Check sheet for the modelled part. Datum: model origin and axes. Units: mm. A direction names the side the tool comes from. Give positions to 0.01 mm unless a question says otherwise; leave off trailing zeros. Write each loop counter-clockwise with the first axis right and the second up, starting at its lowest first coordinate (ties: lowest second). Pieces come first, ordered by that corner, then holes. Notation, with made-up numbers: (36, 79.25) - (94, 79.25) arc R26 ccw to (94, 102.25) - close; hole circle Ø11 at (35, 45.25). An arc over 180 degrees is marked (long way). Return JSON: item names as keys, results as strings. Group by question number.
```python
from build123d import *

# Parameters (mm, degrees)
ESQUISSE1_W        = 29.5
ESQUISSE1_H        = 13
BOSS_EXTRU_2_DEPTH = 7.2
ESQUISSE2_W        = 29.5
ESQUISSE2_H        = 8.4
BOSS_EXTRU_3_DEPTH = 4.3
ESQUISSE4_W        = 7.5
ESQUISSE4_H        = 7.2
BOSS_EXTRU_4_DEPTH = 2
ESQUISSE8_W        = 10.1
ESQUISSE8_H        = 5.9
BOSS_EXTRU_5_DEPTH = 1.2
BOSS_EXTRU_6_START = -10.1
BOSS_EXTRU_6_DEPTH = 10.1
ESQUISSE10_R       = 1.6
BOSS_EXTRU_8_DEPTH = 2


with BuildPart() as part:
    # Esquisse1 → Boss.-Extru.2 (new body)
    with BuildSketch(Plane.XY):
        Rectangle(ESQUISSE1_W, ESQUISSE1_H)
    extrude(amount=BOSS_EXTRU_2_DEPTH)

    # Esquisse2 → Boss.-Extru.3 (add)
    with BuildSketch(Plane.XY.offset(7.2)):
        Rectangle(ESQUISSE2_W, ESQUISSE2_H)
    extrude(amount=BOSS_EXTRU_3_DEPTH)

    # Esquisse4 → Boss.-Extru.4 (add)
    with BuildSketch(Plane.XY.offset(11.5)):
        with Locations((-10.25, 0)):
            Rectangle(ESQUISSE4_W, ESQUISSE4_H)
    extrude(amount=BOSS_EXTRU_4_DEPTH)

    # Esquisse8 → Boss.-Extru.5 (add)
    with BuildSketch(Plane.XY.offset(3.3)):
        with Locations((0, -9.45)):
            Rectangle(ESQUISSE8_W, ESQUISSE8_H)
    extrude(amount=BOSS_EXTRU_5_DEPTH)

    # Esquisse9 → Boss.-Extru.6 (add)
    with BuildSketch(Plane(origin=(5.05, 0, 0), x_dir=(0, 0, -1), z_dir=(1, 0, 0)).offset(BOSS_EXTRU_6_START)):
        Polygon((-4.5, -12.4), (-10.0771346, -12.4), (-10.0771346, -6.830479263), (-8.508865165, -6.830479263), (-7.2, -5.960264638), (-7.2, -6.5), (-4.5, -6.5), align=None)
    extrude(amount=BOSS_EXTRU_6_DEPTH)

    # Esquisse10 → Boss.-Extru.8 (add)
    with BuildSketch(Plane.XY):
        with BuildLine():
            Line((18.5, 3.75), (14.75, 3.75))
            Line((14.75, 3.75), (14.75, 0))
            Line((14.75, 0), (14.75, -3.75))
            Line((14.75, -3.75), (18.5, -3.75))
            ThreePointArc((18.5, -3.75), (22.25, 0), (18.5, 3.75))
        make_face()
        with Locations((18.5, 0)):
            Circle(ESQUISSE10_R, mode=Mode.SUBTRACT)
        with BuildLine():
            Line((-18.5, -3.75), (-14.75, -3.75))
            Line((-14.75, -3.75), (-14.75, 0))
            Line((-14.75, 0), (-14.75, 3.75))
            Line((-14.75, 3.75), (-18.5, 3.75))
            ThreePointArc((-18.5, 3.75), (-22.25, 0), (-18.5, -3.75))
        make_face()
        with Locations((-18.5, 0)):
            Circle(ESQUISSE10_R, mode=Mode.SUBTRACT)
    extrude(amount=BOSS_EXTRU_8_DEPTH)


solid = part.part
```
Item 1: Section check A-A on y = 0. Record the cut outline in (x, z), plus the area to 3 significant figures.
Item 2: Section check D-D on z = 10.75. Record the cut outline in (x, y).
Item 3: Mould release check, pull along Y, two halves, no side actions. Record for faces 1 (the face through (-17, -1, 2)), 2 (the face through (0, -4.2, 9)), 3 (the face through (-22.25, 0.08, 0.99)): +Y half, -Y half, draft (parallel to the pull), parting line (faces both ways), or undercut.
Item 4: Depth check by flat-ended pin: pin 1 (10 mm diameter, centred on x = 9.5, y = 0, fed in from +Z); pin 2 (1.3 mm diameter, centred on x = -2, z = 9.5, fed in from +Y); pin 3 (7 mm diameter, centred on y = -8.5, z = 8, fed in from +X); pin 4 (1.5 mm diameter, centred on x = -16, z = 5, fed in from +Y). Enter the tip coordinate at first touch or a pass-through.
Item 5: Section check C-C on x = -9. Record the cut outline in (y, z), plus the area to 3 significant figures.
Item 6: Access from +Z, -Z, +X, -X, +Y, -Y to the whole of each face (thin tool, end or side, straight path). Record for faces 4 (the face through (-17, 3.75, 1)), 5 (the face through (17, 3.75, 1)), 6 (the face through (0, -10, 10.077)), 7 (the face through (-17, -3.75, 1)).
Item 7: Section check B-B on x = 17.5. Record the cut outline in (y, z).
Item 8: Material ranges on line 1 along Y through (x, z) = (18.5, 0.85); line 2 along X through (y, z) = (3.25, 8.5), recorded low to high. Write a range as from..to.
Reply:
{
 "1": {"outline": "(-22.25, 0) - (-20.1, 0) - (-20.1, 2) - (-22.25, 2) - close; (-16.9, 0) - (16.9, 0) - (16.9, 2) - (14.75, 2) - (14.75, 11.5) - (-6.5, 11.5) - (-6.5, 13.5) - (-14, 13.5) - (-14, 11.5) - (-14.75, 11.5) - (-14.75, 2) - (-16.9, 2) - close; (20.1, 0) - (22.25, 0) - (22.25, 2) - (20.1, 2) - close", "area": "371 mm²"},
 "2": {"outline": "(-14.75, -4.2) - (14.75, -4.2) - (14.75, 4.2) - (-14.75, 4.2) - close"},
 "3": {"face 1": "draft", "face 2": "undercut", "face 3": "parting line"},
 "4": {"pin 1": "z = 11.5", "pin 2": "y = 4.2", "pin 3": "x = 14.75", "pin 4": "through"},
 "5": {"outline": "(-6.5, 0) - (6.5, 0) - (6.5, 7.2) - (4.2, 7.2) - (4.2, 11.5) - (3.6, 11.5) - (3.6, 13.5) - (-3.6, 13.5) - (-3.6, 11.5) - (-4.2, 11.5) - (-4.2, 7.2) - (-6.5, 7.2) - close", "area": "144 mm²"},
 "6": {"face 4": "+Z, -Z, -X, +Y", "face 5": "+Z, -Z, +X, +Y", "face 6": "+Z, +X, -X, -Y", "face 7": "+Z, -Z, -X, -Y"},
 "7": {"outline": "(-3.75, 0) - (-1.25, 0) - (-1.25, 2) - (-3.75, 2) - close; (1.25, 0) - (3.75, 0) - (3.75, 2) - (1.25, 2) - close"},
 "8": {"line 1": "-3.75..-1.6, 1.6..3.75", "line 2": "-14.75..14.75"}
}
